from build123d import *

# Parameters (mm, degrees)
F0_R     = 3.175
F1_DEPTH = 6.35
F3_DEPTH = 0.635


with BuildPart() as f1:
    # F0 (on Top) → F1 (new body)
    with BuildSketch(Plane.XY):
        with BuildLine():
            Line((-6.243237, 5.348631), (-6.107624, 5.161976))
            ThreePointArc((-6.107624, 5.161976), (-6.472362, 4.696551), (-6.801712, 4.205447))
            Line((-6.801712, 4.205447), (-7.01898, 4.276041))
            Line((-7.01898, 4.276041), (-8.536659, 4.769165))
            Line((-8.536659, 4.769165), (-9.710663, 1.150007))
            Line((-9.710663, 1.150007), (-8.194731, 0.657451))
            Line((-8.194731, 0.657451), (-7.975305, 0.586155))
            ThreePointArc((-7.975305, 0.586155), (-7.996815, -0.004769), (-7.9746, -0.595668))
            Line((-7.9746, -0.595668), (-8.191868, -0.666263))
            Line((-8.191868, -0.666263), (-9.709547, -1.159387))
            Line((-9.709547, -1.159387), (-8.532048, -4.777409))
            Line((-8.532048, -4.777409), (-7.016117, -4.284853))
            Line((-7.016117, -4.284853), (-6.796691, -4.213557))
            ThreePointArc((-6.796691, -4.213557), (-6.466756, -4.704268), (-6.101462, -5.169258))
            Line((-6.101462, -5.169258), (-6.235741, -5.354077))
            Line((-6.235741, -5.354077), (-7.173718, -6.645092))
            Line((-7.173718, -6.645092), (-4.094482, -8.880017))
            Line((-4.094482, -8.880017), (-3.157584, -7.590489))
            Line((-3.157584, -7.590489), (-3.021972, -7.403834))
            ThreePointArc((-3.021972, -7.403834), (-2.466616, -7.606897), (-1.897773, -7.768367))
            Line((-1.897773, -7.768367), (-1.897773, -7.996816))
            Line((-1.897773, -7.996816), (-1.897773, -9.592598))
            Line((-1.897773, -9.592598), (1.907038, -9.590761))
            Line((1.907038, -9.590761), (1.907038, -7.996816))
            Line((1.907038, -7.996816), (1.907038, -7.766098))
            ThreePointArc((1.907038, -7.766098), (2.475688, -7.603949), (3.030801, -7.400224))
            Line((3.030801, -7.400224), (3.16508, -7.585043))
            Line((3.16508, -7.585043), (4.103057, -8.876058))
            Line((4.103057, -8.876058), (7.180134, -6.63816))
            Line((7.180134, -6.63816), (6.243237, -5.348631))
            Line((6.243237, -5.348631), (6.107624, -5.161976))
            ThreePointArc((6.107624, -5.161976), (6.472362, -4.696551), (6.801712, -4.205447))
            Line((6.801712, -4.205447), (7.01898, -4.276041))
            Line((7.01898, -4.276041), (8.536659, -4.769165))
            Line((8.536659, -4.769165), (9.710663, -1.150007))
            Line((9.710663, -1.150007), (8.194731, -0.657451))
            Line((8.194731, -0.657451), (7.975305, -0.586155))
            ThreePointArc((7.975305, -0.586155), (7.996815, 0.004769), (7.9746, 0.595668))
            Line((7.9746, 0.595668), (8.191868, 0.666263))
            Line((8.191868, 0.666263), (9.709547, 1.159387))
            Line((9.709547, 1.159387), (8.532048, 4.777409))
            Line((8.532048, 4.777409), (7.016117, 4.284853))
            Line((7.016117, 4.284853), (6.796691, 4.213557))
            ThreePointArc((6.796691, 4.213557), (6.466756, 4.704268), (6.101462, 5.169258))
            Line((6.101462, 5.169258), (6.235741, 5.354077))
            Line((6.235741, 5.354077), (7.173718, 6.645092))
            Line((7.173718, 6.645092), (4.094482, 8.880017))
            Line((4.094482, 8.880017), (3.157584, 7.590489))
            Line((3.157584, 7.590489), (3.021972, 7.403834))
            ThreePointArc((3.021972, 7.403834), (2.466616, 7.606897), (1.897773, 7.768367))
            Line((1.897773, 7.768367), (1.897773, 7.996816))
            Line((1.897773, 7.996816), (1.897773, 9.592598))
            Line((1.897773, 9.592598), (-1.907038, 9.590761))
            Line((-1.907038, 9.590761), (-1.907038, 7.996816))
            Line((-1.907038, 7.996816), (-1.907038, 7.766098))
            ThreePointArc((-1.907038, 7.766098), (-2.475688, 7.603949), (-3.030801, 7.400224))
            Line((-3.030801, 7.400224), (-3.16508, 7.585043))
            Line((-3.16508, 7.585043), (-4.103057, 8.876058))
            Line((-4.103057, 8.876058), (-7.180134, 6.63816))
            Line((-7.180134, 6.63816), (-6.243237, 5.348631))
        make_face()
        Circle(F0_R, mode=Mode.SUBTRACT)
    extrude(amount=F1_DEPTH)

    # F2 (on face) → F3 (join)
    with BuildSketch(Plane.XY.offset(6.35)):
        Polygon((-2.151463, 6.638584), (-3.030801, 6.63816), (-1.354291, 3.640304), (-0.13337, 5.854254), (1.136369, 5.854867), (0.194719, 3.640106), (1.091522, 3.640106), (2.033314, 5.855201), (3.169588, 5.85575), (3.602625, 6.640995), (2.839816, 6.640995), (0.299816, 6.639768), (-0.577028, 6.639345), (-1.358951, 5.221451), align=None)
        Polygon((-2.288674, -3.76517), (-3.168012, -3.765595), (-1.491502, -6.763451), (-0.27058, -4.549501), (0.999159, -4.548888), (0.057508, -6.763649), (0.954311, -6.763649), (1.896103, -4.548553), (3.032377, -4.548005), (3.465414, -3.76276), (2.702605, -3.76276), (0.162605, -3.763986), (-0.714239, -3.76441), (-1.496161, -5.182303), align=None)
    extrude(amount=F3_DEPTH)


solid = f1.part
Here's how the part is built. I have some questions about the finished solid (model axes, mm). A direction names the side the tool comes from. Give positions to 0.01 mm unless a question says otherwise; leave off trailing zeros. Order: outer loops, then holes, each group sorted by start corner. A loop starts at its lowest first (then second) coordinate and runs counter-clockwise, first axis right, second up. Notation, with made-up numbers: (6.5, 3.25) -> (15.5, 3.25) arc R26 cw to (15.5, 30.25) -> close; hole circle Ø1 at (56, -27.5). An arc over 180 degrees is marked (long way). Use a Markdown table: item, result. Add a question column.
Item 1: Imagine slicing it at C-C on x = -7.5. Please give me the cut outline in (y, z), plus the area to 3 significant figures.
Item 2: Imagine slicing it at B-B on x = 5.5. Please give me the cut outline in (y, z).
Item 3: Imagine slicing it at A-A on y = 0. Please give me the cut outline in (x, z) (3 decimals), plus the area to 3 significant figures.
Item 4: If we mould it in two halves opening along Y, with no side actions, what happens to faces 6 (the face through (2.468, -7.607, 3.131)), 7 (the face through (6.47, 4.7, 3.13)), 8 (the face through (-1.907, 9, 3)), 9 (the face through (-9.115, 2.985, 3.131))? For each: pulls with the +Y half, pulls with the -Y half, needs draft (parallel to the pull), parting line crosses it, or undercut.
Item 5: Will these pins go through, and if not, where does the flat tip stop? pin 1 (0.9 mm diameter, centred on y = -8.5, z = 4.5, fed in from +X); pin 2 (1.5 mm diameter, centred on x = 6, z = 2, fed in from -Y); pin 3 (1 mm diameter, centred on x = -4, z = 5, fed in from -Y).
Item 6: For faces 1 (the face through (-2.204, 5.16, 6.663)), 2 (the face through (1.898, 9, 3)), 3 (the face through (-6.47, 4.7, 3.13)), 4 (the face through (-0.89, -5.67, 6.66)), 5 (the face through (0.67, 4.76, 6.66)), which set-ups out of +Z, -Z, +X, -X, +Y, -Y let a thin tool reach every point of the face, with its end or its side?
Item 7: I need wall thicknesses on line 1 (Y direction, x = 0, z = 5) (3 decimals); line 2 (Z direction, x = 6.25, y = 1.5); line 3 (X direction, y = 8.75, z = 2.75). Which ranges of each line are inside material? Lowest first, please.
Data:
| question | item | result |
|---|---|---|
| 1 | outline | (-4.44, 0) -> (4.43, 0) -> (4.43, 6.35) -> (-4.44, 6.35) -> close |
| 1 | area | 56.4 mm² |
| 2 | outline | (-7.86, 0) -> (7.86, 0) -> (7.86, 6.35) -> (-7.86, 6.35) -> close |
| 3 | outline | (-7.997, 0) -> (-3.175, 0) -> (-3.175, 6.35) -> (-7.997, 6.35) -> close; (3.175, 0) -> (7.997, 0) -> (7.997, 6.35) -> (3.175, 6.35) -> close |
| 3 | area | 61.2 mm² |
| 4 | face 6 | pulls with the -Y half |
| 4 | face 7 | undercut |
| 4 | face 8 | needs draft |
| 4 | face 9 | pulls with the +Y half |
| 5 | pin 1 | stops at x = 5.24 |
| 5 | pin 2 | stops at y = -8.04 |
| 5 | pin 3 | stops at y = -8.88 |
| 6 | face 1 | +Z, -X |
| 6 | face 2 | +Z, -Z, +Y |
| 6 | face 3 | +Z, -Z |
| 6 | face 4 | +Z, -Y |
| 6 | face 5 | +Z |
| 7 | line 1 | y = -9.592 to -3.175, 3.175 to 9.592 |
| 7 | line 2 | z = 0 to 6.35 |
| 7 | line 3 | x = -4.28 to -4.01, -1.91 to 1.9, 4 to 4.27 |
